CAD build for the part. Positions are in the model's coordinates, mm. A direction names the side the tool comes from. Coordinates: 2 decimals unless noted, no trailing zeros. Loops run counter-clockwise (first coordinate to the right, second up) from the corner with the lowest first, then second, coordinate; pieces in that order, holes last. Notation, with made-up numbers: (55, 32.5) -> (101, 32.5) arc R12 ccw to (101, 41.5) -> close; hole circle Ø4 at (59, 49). An arc over 180 degrees is marked (long way). Write item = value, one per line. Start each with the question number.
(1) Pull direction Z, two halves, no side cores. Call faces 4 (the face through (-32.194, 0, 62)), 5 (the face through (0, -30.924, 34)), 6 (the face through (-8, 0, 0)): +Z half, -Z half, draft (parallel to the pull), parting line (faces both ways), or undercut.
(2) Band-saw the part on A-A (x = 0). Write the cut outline in (y, z) (1 decimal).
(3) Tool access for faces 1 (the face through (24, 27.75, 46)), 2 (the face through (-16, 30.924, 51)), 3 (the face through (32.194, 0, 62)): list every direction of +Z, -Z, +X, -X, +Y, -Y with a clear straight run to the whole face (end or side of a thin tool).
(4) Flat gauge pins, fed straight in: P1, Ø3, axis at x = 11, y = -7.5, coming from the +Z side; P2, Ø1, axis at x = -31.5, z = 63.5, coming from the +Y side; P3, Ø5, axis at y = 11.5, z = 63.5, coming from the -X side. Where does each tip first touch, or does it go through?
(5) Drill centre lines: line 1 (X direction, y = 0, z = 49.5); line 2 (X direction, y = -3.5, z = 62.5). Where is each one in solid material? Low to high. Write a range as from..to.
(6) Band-saw the part on B-B (z = 9). Write the cut outline in (x, y) (1 decimal), and give its area (3 significant figures).
```python
from build123d import *

# Parameters (mm, degrees)
F0_W      = 68.199
F0_H      = 68.199
F1_DEPTH  = 66.6115
F2_R      = 1.5875
F3_T      = -3.175
F4_W      = 3.175
F4_H      = 3.175
F4_W_2    = 6.35
F4_H_2    = 6.35
F5_DEPTH  = 25.4
F6_R      = 1.5875
F7_DEPTH  = 6.35
F8_W      = 74.20966
F8_H      = 75.78341
F9_DEPTH  = 6.35
F10_W     = 6.35
F10_H     = 1.5875
F11_DEPTH = 66.295
F12_W     = 6.35
F12_H     = 1.5875
F13_DEPTH = 66.295
F14_R     = 10.00125
F14_R_2   = 9.2075
F15_DEPTH = 61.849
F16_W     = 55.499
F16_H     = 55.499
F17_DEPTH = 38.1
F18_W     = 61.849
F18_H     = 61.849
F19_DEPTH = 0.79375
F20_W     = 68.199
F20_H     = 68.199
F21_DEPTH = 66.6125


with BuildPart() as f1:
    # F0 (on Top) → F1 (new body)
    with BuildSketch(Plane.XY):
        Rectangle(F0_W, F0_H)
    extrude(amount=F1_DEPTH)

    # F2
    f2_edges = [f1.edges().sort_by_distance(p)[0] for p in [
        (-34.0995, 34.0995, 33.30575),
        (-34.0995, 0, 0),
        (-34.0995, -34.0995, 33.30575),
        (34.0995, -34.0995, 33.30575),
        (0, -34.0995, 0),
        (34.0995, 0, 0),
        (0, 34.0995, 0),
        (34.0995, 34.0995, 33.30575),
    ]]
    fillet(f2_edges, radius=F2_R)

    # F3
    f3_openings = [f1.faces().sort_by_distance(p)[0] for p in [
        (0, 0, 66.6115),
    ]]
    offset(amount=F3_T, openings=f3_openings)

    # F4 (on face) → F5 (cut)
    with BuildSketch(Plane.XY.offset(3.175)):
        with Locations((-29.337, 29.337)):
            Rectangle(F4_W, F4_H)
        with Locations((29.337, 29.337)):
            Rectangle(F4_W, F4_H)
        with Locations((-29.337, -29.337)):
            Rectangle(F4_W, F4_H)
        with Locations((29.337, -29.337)):
            Rectangle(F4_W, F4_H)
        with Locations((0, 29.337)):
            Rectangle(F4_W_2, F4_H)
        with Locations((-29.337, 0)):
            Rectangle(F4_W, F4_H_2)
        with Locations((29.337, 0)):
            Rectangle(F4_W, F4_H_2)
        with Locations((0, -29.337)):
            Rectangle(F4_W_2, F4_H)
    extrude(amount=F5_DEPTH, mode=Mode.SUBTRACT)

    # F6 (on face) → F7 (cut)
    with BuildSketch(Plane(origin=(0, 0, 0), x_dir=(1, 0, 0), z_dir=(0, 0, -1))):
        Circle(F6_R)
    extrude(amount=-F7_DEPTH, mode=Mode.SUBTRACT)

    # F8 (on face) → F9 (cut)
    with BuildSketch(Plane.XY.offset(66.6115)):
        Rectangle(F8_W, F8_H)
        with BuildLine():
            Line((-30.607, 32.1945), (30.607, 32.1945))
            ThreePointArc((30.607, 32.1945), (31.729532, 31.729532), (32.1945, 30.607))
            Line((32.1945, 30.607), (32.1945, -30.607))
            ThreePointArc((32.1945, -30.607), (31.729532, -31.729532), (30.607, -32.1945))
            Line((30.607, -32.1945), (-30.607, -32.1945))
            ThreePointArc((-30.607, -32.1945), (-31.729532, -31.729532), (-32.1945, -30.607))
            Line((-32.1945, -30.607), (-32.1945, 30.607))
            ThreePointArc((-32.1945, 30.607), (-31.729532, 31.729532), (-30.607, 32.1945))
        make_face(mode=Mode.SUBTRACT)
    extrude(amount=-F9_DEPTH, mode=Mode.SUBTRACT)

    # F10 (on face) → F11 (cut, through all)
    with BuildSketch(Plane.XZ.offset(32.1945)):
        with Locations((0, 63.4365)):
            Rectangle(F10_W, F10_H)
    extrude(amount=-F11_DEPTH, mode=Mode.SUBTRACT)

    # F12 (on face) → F13 (cut, through all)
    with BuildSketch(Plane.YZ.offset(32.1945)):
        with Locations((0, 63.4365)):
            Rectangle(F12_W, F12_H)
    extrude(amount=-F13_DEPTH, mode=Mode.SUBTRACT)

    # F14 (on face) → F15 (join, through all)
    with BuildSketch(Plane.XZ.offset(-30.9245)):
        with Locations((-15.875, 50.8)):
            Circle(F14_R)
        with Locations((-15.875, 50.8)):
            Circle(F14_R_2, mode=Mode.SUBTRACT)
        with Locations((15.875, 50.8)):
            Circle(F14_R)
        with Locations((15.875, 50.8)):
            Circle(F14_R_2, mode=Mode.SUBTRACT)
    extrude(amount=F15_DEPTH)

    # F16 (on face) → F17 (cut)
    with BuildSketch(Plane.XY.offset(66.6115)):
        Rectangle(F16_W, F16_H)
    extrude(amount=-F17_DEPTH, mode=Mode.SUBTRACT)

    # F18 (on face) → F19 (cut)
    with BuildSketch(Plane.XY.offset(3.175)):
        Rectangle(F18_W, F18_H)
    extrude(amount=-F19_DEPTH, mode=Mode.SUBTRACT)

    # F20 (on face) → F21 (cut, through all)
    with BuildSketch(Plane.XY.offset(66.6115)):
        Rectangle(F20_W, F20_H)
        with BuildLine():
            Line((-31.6865, 33.274), (31.6865, 33.274))
            ThreePointArc((31.6865, 33.274), (32.809032, 32.809032), (33.274, 31.6865))
            Line((33.274, 31.6865), (33.274, -31.6865))
            ThreePointArc((33.274, -31.6865), (32.809032, -32.809032), (31.6865, -33.274))
            Line((31.6865, -33.274), (-31.6865, -33.274))
            ThreePointArc((-31.6865, -33.274), (-32.809032, -32.809032), (-33.274, -31.6865))
            Line((-33.274, -31.6865), (-33.274, 31.6865))
            ThreePointArc((-33.274, 31.6865), (-32.809032, 32.809032), (-31.6865, 33.274))
        make_face(mode=Mode.SUBTRACT)
    extrude(amount=-F21_DEPTH, mode=Mode.SUBTRACT)


solid = f1.part
```
Findings below:
q1.face_4 = draft
q1.face_5 = undercut
q1.face_6 = -Z half
q2.outline = (-33.3, 0.2) arc R1.6 ccw to (-32.5, 0) -> (-1.6, 0) -> (-1.6, 2.4) -> (-30.9, 2.4) -> (-30.9, 62.6) -> (-32.2, 62.6) -> (-32.2, 60.3) -> (-33.3, 60.3) -> close; (-32.2, 64.2) -> (-30.9, 64.2) -> (-30.9, 66.6) -> (-32.2, 66.6) -> close; (1.6, 0) -> (32.5, 0) arc R1.6 ccw to (33.3, 0.2) -> (33.3, 60.3) -> (32.2, 60.3) -> (32.2, 62.6) -> (30.9, 62.6) -> (30.9, 2.4) -> (1.6, 2.4) -> close; (30.9, 64.2) -> (32.2, 64.2) -> (32.2, 66.6) -> (30.9, 66.6) -> close
q3.face_1 = +Z
q3.face_2 = none
q3.face_3 = +Z, +X, +Y, -Y
q4.P1 = 2.38
q4.P2 = 32.15
q4.P3 = -32.19
q5.line_1 = -33.27..-30.92, 30.92..33.27
q5.line_2 = -32.19..-30.92, 30.92..32.19
q6.outline = (-33.3, -31.7) arc R1.6 ccw to (-31.7, -33.3) -> (31.7, -33.3) arc R1.6 ccw to (33.3, -31.7) -> (33.3, 31.7) arc R1.6 ccw to (31.7, 33.3) -> (-31.7, 33.3) arc R1.6 ccw to (-33.3, 31.7) -> close; hole (-30.9, -30.9) -> (30.9, -30.9) -> (30.9, 30.9) -> (-30.9, 30.9) -> close
q6.area = 601 mm²
